Geometry check sheet. Reference: the model listing, model coordinates, mm. A direction names the side the tool comes from. Give positions to 0.01 mm unless a question says otherwise; leave off trailing zeros. Loops run counter-clockwise (first coordinate to the right, second up) from the corner with the lowest first, then second, coordinate; pieces in that order, holes last.
1. Cross-section at A-A, the plane z = 0. Record the cut outline in (x, y), plus the area to 3 significant figures.
2. Tool access check on faces 1 (the flat face through (-31.091, -13, 45)), 2 (the flat face through (31.084, -13, 44)), 3 (the cylindrical face through (-4.6, 49.733, -30.896)), 4 (the cylindrical face through (-3.045, 51.867, -13.714)). Record the directions out of +Z, -Z, +X, -X, +Y, -Y that give a thin tool (end or side, any length) a straight path to the whole face; none if there is none.
3. Release check for a two-part mould opening along Y. For faces 5 (the cylindrical face through (-3.03, -12.88, 71.96)), 6 (the flat face through (0, -25.4, 44)), 7 (the flat face through (0, 101.6, 61)) record: +Y half, -Y half, draft (parallel to the pull), parting line (faces both ways), or undercut.
4. Go/stop test with flat-tipped pins: pin 1 Ø12.5 at (y, z) = (-11, 47.5) entering from +X; pin 2 Ø1 at (x, z) = (-12, 3) entering from -Y; pin 3 Ø12 at (x, y) = (-15.5, 42.5) entering from -Z; pin 4 Ø7.5 at (y, z) = (-11, 24.5) entering from -X. Record where each tip stops, or that it passes through.
5. Cross-section at D-D, the plane y = 7. Record the cut outline in (x, z).
6. Cross-section at C-C, the plane y = -9.5. State how many separate pieces and enclosed holes the cut face has, plus the area to 3 significant figures.
7. Material ranges on L1, parallel to Z at x = 0, y = -7; L2, parallel to Z at x = 0, y = 40.5; L3, parallel to Y at x = -13, z = 32, recorded low to high.
8. Cross-section at B-B, the plane x = 0. Record the cut outline in (y, z), plus the area to 3 significant figures.
from build123d import *

# Parameters (mm, degrees)
F0_R      = 31.236454
F2_DEPTH  = 25.4
F3_DEPTH  = 25.4
F4_DEPTH  = 50.8
F5_R      = 14.047882
F6_DEPTH  = 76.201
F8_W      = 31.083973
F8_H      = 25.4
F10_W     = 31.09123
F10_H     = 25.4
F12_R     = 13.98371
F13_DEPTH = 152.401


with BuildPart() as f2:
    # F0 (on Front) → F2 (new body)
    with BuildSketch(Plane.XZ):
        Circle(F0_R)
    extrude(amount=F2_DEPTH)

    # F1 (on face) → F3 (join)
    with BuildSketch(Plane.XZ):
        with BuildLine():
            Line((0, 85.611142), (0, 31.236454))
            ThreePointArc((0, 31.236454), (20.969327, 23.151746), (31.083973, 3.082637))
            Line((31.083973, 3.082637), (31.083973, 85.611142))
            Line((31.083973, 85.611142), (0, 85.611142))
        make_face()
        with BuildLine():
            Line((-31.09123, 85.611142), (-31.09123, 3.008564))
            ThreePointArc((-31.09123, 3.008564), (-20.996895, 23.126747), (0, 31.236454))
            Line((0, 31.236454), (0, 85.611142))
            Line((0, 85.611142), (-31.09123, 85.611142))
        make_face()
    extrude(amount=F3_DEPTH)

    # F0 (on Front) → F4 (join)
    with BuildSketch(Plane.XZ):
        Circle(F0_R)
    extrude(amount=-F4_DEPTH)

    # F5 (on face) → F6 (cut, through all)
    with BuildSketch(Plane.XZ.offset(25.4)):
        Circle(F5_R)
    extrude(amount=-F6_DEPTH, mode=Mode.SUBTRACT)

    # F7: F2 across face


with BuildPart() as f2_1:
    add(f2.part)
    add(f2.part.mirror(Plane(origin=(0, 50.8, 0), x_dir=(1, 0, 0), z_dir=(0, 1, 0))))

    # F8 (on face) → F9 (revolve)
    with BuildSketch(Plane.XY.offset(85.611142)):
        with Locations((15.541987, -12.7)):
            Rectangle(F8_W, F8_H)
    revolve(axis=Axis((0, -12.7, 85.611142), (0, -1, 0)))

    # F10 (on face) → F11 (revolve)
    with BuildSketch(Plane.XY.offset(85.611142)):
        with Locations((-15.545615, 114.3)):
            Rectangle(F10_W, F10_H)
    revolve(axis=Axis((0, 114.3, 85.611142), (0, 1, 0)))

    # F12 (on face) → F13 (cut, through all)
    with BuildSketch(Plane.XZ.offset(25.4)):
        with Locations((0, 85.611142)):
            Circle(F12_R)
    extrude(amount=-F13_DEPTH, mode=Mode.SUBTRACT)


solid = f2_1.part
Result:
1. outline: (-31.24, -25.4) - (-14.05, -25.4) - (-14.05, 127) - (-31.24, 127) - close; (14.05, -25.4) - (31.24, -25.4) - (31.24, 127) - (14.05, 127) - close
1. area: 5,240 mm2
2. face 1: +Z, -X, +Y, -Y
2. face 2: +Z, +X, +Y, -Y
2. face 3: none
2. face 4: +Y, -Y
3. face 5: draft
3. face 6: -Y half
3. face 7: undercut
4. pin 1: stops at x = 31.08
4. pin 2: passes through
4. pin 3: stops at z = -29.76
4. pin 4: stops at x = -31.09
5. outline: circle Ø62.47 at (0, 0); hole circle Ø28.1 at (0, 0)
6. separate pieces: 1
6. enclosed holes: 2
6. area: 7,140 mm2
7. L1: z = -31.24 to -14.05, 14.05 to 71.63, 99.59 to 116.7
7. L2: z = -31.24 to -14.05, 14.05 to 31.24
7. L3: y = -25.4 to 0, 101.6 to 127
8. outline: (-25.4, -31.24) - (127, -31.24) - (127, -14.05) - (-25.4, -14.05) - close; (-25.4, 14.05) - (127, 14.05) - (127, 71.63) - (101.6, 71.63) - (101.6, 31.24) - (0, 31.24) - (0, 71.63) - (-25.4, 71.63) - close; (-25.4, 99.59) - (0, 99.59) - (0, 116.7) - (-25.4, 116.7) - close; (101.6, 99.59) - (127, 99.59) - (127, 116.7) - (101.6, 116.7) - close
8. area: 8,160 mm2
